The figure shows three views and two pictorial views of one solid part (mm, origin at its lowest corner). Answer the questions. A direction names the side the tool comes from. Round coordinates to 2 decimals unless told otherwise and drop trailing zeros. Write each loop counter-clockwise with the first axis right and the second up, starting at its lowest first coordinate (ties: lowest second). Pieces come first, ordered by that corner, then holes.
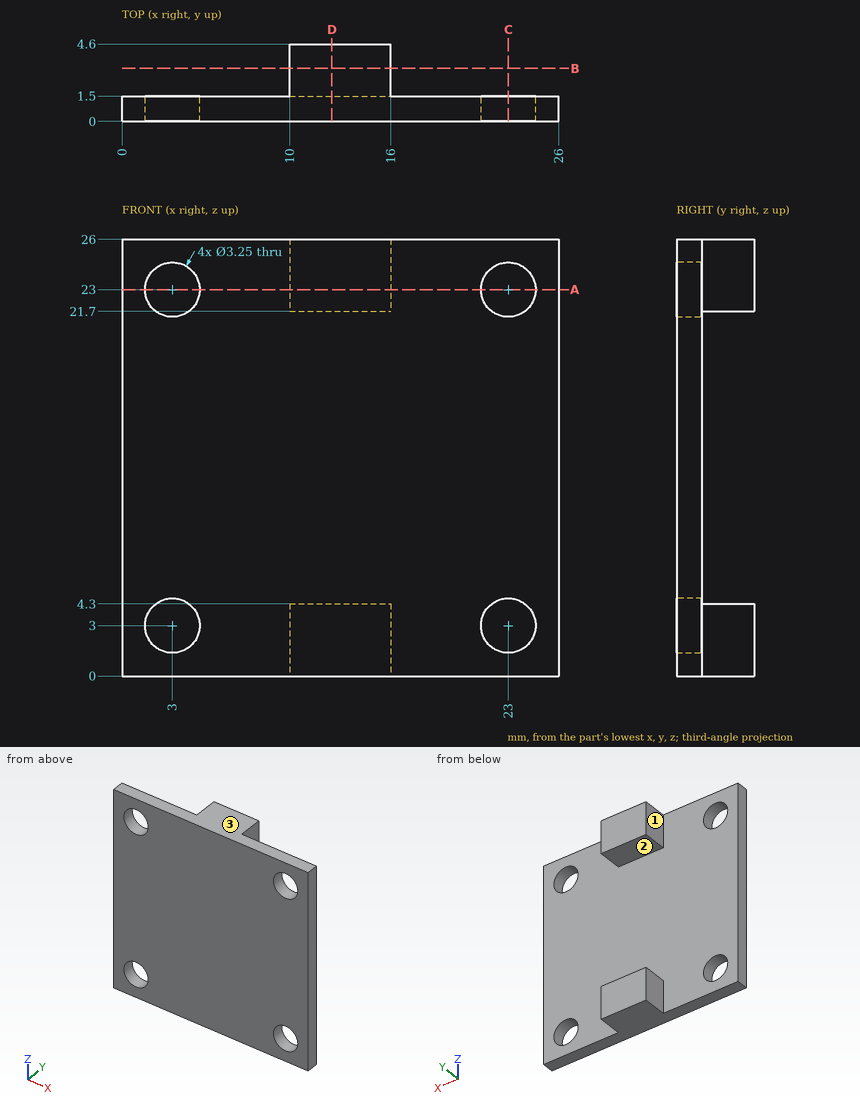
Q1. Section D-D (x = 12.5) is taken. Determine the outline of the cut face in (y, z), then the cut area to 3 significant figures.
Verdict:
outline: (0, 0) - (4.6, 0) - (4.6, 4.3) - (1.5, 4.3) - (1.5, 21.7) - (4.6, 21.7) - (4.6, 26) - (0, 26) - close
area: 65.7 mm2
Q2. Which of the six approach directions +Z, -Z, +X, -X, +Y, -Y give full straight-line access (tool end or side, diameter ignored) to the marked faces 1, 2 and 3?
Verdict:
face 1: +Z, -Z, -X, +Y
face 2: +X, -X, +Y
face 3: +Z, +X, -X, +Y, -Y
Q3. Flat-ended cylindrical pins translate along their axes: pin 1 Ø1.5 at (y, z) = (3.5, 23.5) entering from +X; pin 2 Ø4 at (x, z) = (23, 3) entering from +Y; pin 3 Ø2.5 at (y, z) = (3.5, 23.5) entering from -X. Find the tip coordinate at first contact, or state that the pin passes through.
Verdict:
pin 1: stops at x = 16
pin 2: stops at y = 1.5
pin 3: stops at x = 10
Q4. Straight lines are drawn through the part: probe 1 along X at (y, z) = (1.4, 3) (3 decimals); probe 2 along Z at (x, y) = (14, 1.7); probe 3 along Y at (x, z) = (18.5, 3.75). For each, find the intervals that lie inside material, in ascending order.
Verdict:
probe 1: x = 0 to 1.375, 4.625 to 21.375, 24.625 to 26
probe 2: z = 0 to 4.3, 21.7 to 26
probe 3: y = 0 to 1.5
Q5. Section B-B (y = 3.15) is taken. Determine the outline of the cut face in (x, z).
Verdict:
outline: (10, 0) - (16, 0) - (16, 4.3) - (10, 4.3) - close; (10, 21.7) - (16, 21.7) - (16, 26) - (10, 26) - close
Q6. Section C-C (x = 23) is taken. Determine the outline of the cut face in (y, z) (3 decimals), then the cut area to 4 significant figures.
Verdict:
outline: (0, 0) - (1.5, 0) - (1.5, 1.375) - (0, 1.375) - close; (0, 4.625) - (1.5, 4.625) - (1.5, 21.375) - (0, 21.375) - close; (0, 24.625) - (1.5, 24.625) - (1.5, 26) - (0, 26) - close
area: 29.25 mm2
Q7. Section A-A (z = 23) is taken. Determine the outline of the cut face in (x, y) (3 decimals).
Verdict:
outline: (0, 0) - (1.375, 0) - (1.375, 1.5) - (0, 1.5) - close; (4.625, 0) - (21.375, 0) - (21.375, 1.5) - (16, 1.5) - (16, 4.6) - (10, 4.6) - (10, 1.5) - (4.625, 1.5) - close; (24.625, 0) - (26, 0) - (26, 1.5) - (24.625, 1.5) - close
